from build123d import *

# Parameters (mm, degrees)
ESTRUSIONE_ESTRUSIONE1_DEPTH      = 17.5
ESTRUSIONE_ESTRUSIONE1_DEPTH_BACK = 3
SCHIZZO1_W                        = 3
SCHIZZO1_H                        = 37.84787706
SCHIZZO2_W                        = 3
SCHIZZO2_H                        = 42.5
ESTRUSIONE_ESTRUSIONE2_DEPTH      = 5
SCHIZZO3_W                        = 25
SCHIZZO3_H                        = 0.57606147
TAGLIO_ESTRUSIONE1_DEPTH          = 10
RACCORDO1_R                       = 4
RACCORDO1_OF_SPECCHIA1_R          = 4


with BuildPart() as part:
    # Schizzo1 → Estrusione-Estrusione1 (new, two sides: drawn at the far end of the back side and taken through both)
    with BuildSketch(Plane.XY.offset(-ESTRUSIONE_ESTRUSIONE1_DEPTH_BACK)):
        with Locations((-225, 0)):
            Rectangle(SCHIZZO1_W, SCHIZZO1_H)
    extrude(amount=ESTRUSIONE_ESTRUSIONE1_DEPTH + ESTRUSIONE_ESTRUSIONE1_DEPTH_BACK)

    # Schizzo2 → Estrusione-Estrusione2 (add)
    with BuildSketch(Plane(origin=(0, 18.92393853, 0), x_dir=(1, 0, 0), z_dir=(0, 1, 0))):
        with Locations((-225, -21.25)):
            Rectangle(SCHIZZO2_W, SCHIZZO2_H)
    estrusione_estrusione2 = extrude(amount=ESTRUSIONE_ESTRUSIONE2_DEPTH)

    # Schizzo3 → Taglio-Estrusione1 (cut)
    with BuildSketch(Plane(origin=(-223.5, 0, 0), x_dir=(0, 0, -1), z_dir=(1, 0, 0))):
        with Locations((-30, 19.211969265)):
            Rectangle(SCHIZZO3_W, SCHIZZO3_H)
    taglio_estrusione1 = extrude(amount=-TAGLIO_ESTRUSIONE1_DEPTH, mode=Mode.SUBTRACT)

    # Raccordo1
    raccordo1_edges = [part.edges().sort_by_distance(p)[0] for p in [
        (-225, 19.5, 17.5),
    ]]
    fillet(raccordo1_edges, radius=RACCORDO1_R)

    # Specchia1: Estrusione-Estrusione2, Taglio-Estrusione1 across plane
    add(estrusione_estrusione2.mirror(Plane.ZX))
    add(taglio_estrusione1.mirror(Plane.ZX), mode=Mode.SUBTRACT)

    # Raccordo1 of Specchia1
    raccordo1_of_specchia1_edges = [part.edges().sort_by_distance(p)[0] for p in [
        (-225, -19.5, 17.5),
    ]]
    fillet(raccordo1_of_specchia1_edges, radius=RACCORDO1_OF_SPECCHIA1_R)


solid = part.part
Here's how the part is built. I have some questions about the finished solid (model axes, mm). A direction names the side the tool comes from. Round coordinates to 2 decimals unless told otherwise and drop trailing zeros. Write each loop counter-clockwise with the first axis right and the second up, starting at its lowest first coordinate (ties: lowest second). Pieces come first, ordered by that corner, then holes.
1. Suppose I cut it at B-B (x = -225.75). List the corners of the cut face in (y, z) for me, and give its area (3 significant figures).
2. Suppose I cut it at A-A (z = 30.5). List the corners of the cut face in (x, y) for me, and give its area (3 significant figures).
3. Will these pins go through, and if not, where does the flat tip stop? pin 1 Ø0.9 at (x, z) = (-224.5, -2) entering from +Y; pin 2 Ø1.5 at (x, y) = (-225, 21) entering from -Z; pin 3 Ø1 at (x, y) = (-225.5, 4.5) entering from +Z.
4. I need wall thicknesses on L1, parallel to Y at x = -224.35, z = 28.5; L2, parallel to Z at x = -224.3, y = -5.5; L3, parallel to Z at x = -224.9, y = 21. Which ranges of each line are inside material? Lowest first, please.
5. For faces 5 (the flat face through (-225, 21, 0)), 6 (the flat face through (-225, 19.5, 32)), 7 (the flat face through (-225, -21, 0)), which set-ups out of +Z, -Z, +X, -X, +Y, -Y let a thin tool reach every point of the face, with its end or its side?
6. Suppose I cut it at C-C (y = 14). List the corners of the cut face in (x, z) for me, and give its area (3 significant figures).
7. If we mould it in two halves opening along Y, with no side actions, what happens to faces 1 (the flat face through (-225, -18.924, -2)), 2 (the flat face through (-225, -22, 42.5)), 3 (the cylindrical face through (-225.021, -18.297, 18.641)), 4 (the flat face through (-225, 0, 17.5))? For each: released by +Y, released by -Y, zero draft, split by the parting line, or undercut.
8. Suppose I cut it at D-D (y = -17). List the corners of the cut face in (x, z) for me.
Answer sheet:
1. outline: (-23.92, 0) - (-18.92, 0) - (-18.92, -3) - (18.92, -3) - (18.92, 0) - (23.92, 0) - (23.92, 42.5) - (19.5, 42.5) - (19.5, 21.5) arc R4 cw to (15.5, 17.5) - (-15.5, 17.5) arc R4 cw to (-19.5, 21.5) - (-19.5, 42.5) - (-23.92, 42.5) - close
1. area: 1,180 mm2
2. outline: (-226.5, -23.92) - (-223.5, -23.92) - (-223.5, -19.5) - (-226.5, -19.5) - close; (-226.5, 19.5) - (-223.5, 19.5) - (-223.5, 23.92) - (-226.5, 23.92) - close
2. area: 26.5 mm2
3. pin 1: stops at y = 18.92
3. pin 2: stops at z = 0
3. pin 3: stops at z = 17.5
4. L1: y = -23.92 to -19.5, 19.5 to 23.92
4. L2: z = -3 to 17.5
4. L3: z = 0 to 42.5
5. face 5: -Z, +X, -X, +Y
5. face 6: +Z, +X, -X
5. face 7: -Z, +X, -X, -Y
6. outline: (-226.5, -3) - (-223.5, -3) - (-223.5, 17.5) - (-226.5, 17.5) - close
6. area: 61.5 mm2
7. face 1: released by -Y
7. face 2: zero draft
7. face 3: undercut
7. face 4: undercut
8. outline: (-226.5, -3) - (-223.5, -3) - (-223.5, 17.79) - (-226.5, 17.79) - close
